Check sheet for the modelled part. Datum: model origin and axes. Units: mm. Face numbers are marked on the shaded views. A direction names the side the tool comes from. Coordinates: 2 decimals unless noted, no trailing zeros. Order: outer loops, then holes, each group sorted by start corner. A loop starts at its lowest first (then second) coordinate and runs counter-clockwise, first axis right, second up.
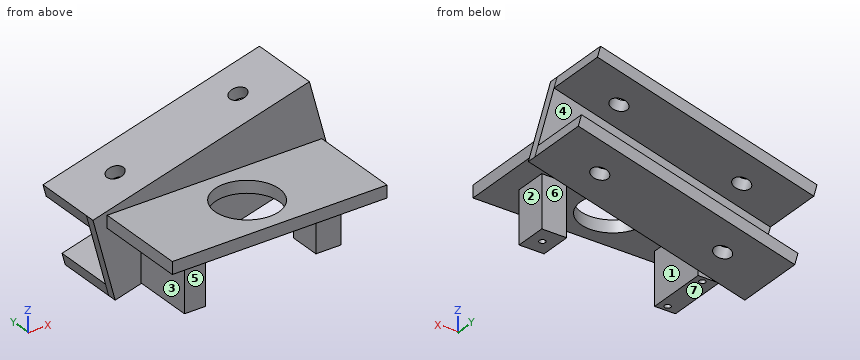
from build123d import *

# Parameters (mm, degrees)
SKETCH1_W           = 70
SKETCH1_H           = 30
SKETCH1_R           = 10.5
BOSS_EXTRUDE1_DEPTH = 4
SKETCH3_W           = 8.150987667
SKETCH3_H           = 10.43538234
SKETCH3_W_2         = 6.820916115
SKETCH3_H_2         = 20
BOSS_EXTRUDE2_DEPTH = 17
SKETCH4_R           = 1
CUT_EXTRUDE1_DEPTH  = 17
BOSS_EXTRUDE4_DEPTH = 3
BOSS_EXTRUDE5_DEPTH = 20
SKETCH10_R          = 2.75
CUT_EXTRUDE2_DEPTH  = 47.267747797


with BuildPart() as part:
    # Sketch1 → Boss-Extrude1 (new body)
    with BuildSketch(Plane.XY):
        with Locations((35, -15)):
            Rectangle(SKETCH1_W, SKETCH1_H)
        with Locations((35, -15)):
            Circle(SKETCH1_R, mode=Mode.SUBTRACT)
    extrude(amount=BOSS_EXTRUDE1_DEPTH)

    # Sketch3 → Boss-Extrude2 (add)
    with BuildSketch(Plane(origin=(0, 0, 0), x_dir=(-1, 0, 0), z_dir=(0, 0, -1))):
        with Locations((-58.424506167, -14.156074174)):
            Rectangle(SKETCH3_W, SKETCH3_H)
        with Locations((-10.910458058, -15)):
            Rectangle(SKETCH3_W_2, SKETCH3_H_2)
    extrude(amount=BOSS_EXTRUDE2_DEPTH)

    # Sketch4 → Cut-Extrude1 (cut)
    with BuildSketch(Plane(origin=(0, 0, -17), x_dir=(-1, 0, 0), z_dir=(0, 0, -1))):
        with Locations((-58.5, -14.289099526)):
            Circle(SKETCH4_R)
        with Locations((-11.5, -7)):
            Circle(SKETCH4_R)
        with Locations((-11.5, -23)):
            Circle(SKETCH4_R)
    extrude(amount=-CUT_EXTRUDE1_DEPTH, mode=Mode.SUBTRACT)

    # Sketch7 → Boss-Extrude4 (add)
    with BuildSketch(Plane(origin=(0, 0, 0), x_dir=(1, 0, 0), z_dir=(0, 1, 0))):
        Polygon((-4.630368757, -4), (65.950788783, -22.912164164), (73.197722046, 4.133758972), (2.616564506, 23.045923136), align=None)
    extrude(amount=BOSS_EXTRUDE4_DEPTH)

    # Sketch9 → Boss-Extrude5 (add)
    with BuildSketch(Plane(origin=(0, 3, 0), x_dir=(1, 0, 0), z_dir=(0, 1, 0))):
        Polygon((-4.630368757, -4), (65.950788783, -22.912164164), (66.943950204, -19.205635281), (-3.595092577, -0.136296695), align=None)
        Polygon((2.616564506, 23.045923136), (1.581288325, 19.182219831), (72.162445865, 0.270055667), (73.197722046, 4.133758972), align=None)
    extrude(amount=BOSS_EXTRUDE5_DEPTH)

    # Sketch10 → Cut-Extrude2 (cut, through all)
    with BuildSketch(Plane(origin=(5.936757371, 0, -22.156280139), x_dir=(-0.965925826, 0, -0.258819045), z_dir=(0.258819045, 0, -0.965925826))):
        with Locations((-53.953749554, 11.5)):
            Circle(SKETCH10_R)
        with Locations((-12.488324975, 11.5)):
            Circle(SKETCH10_R)
    extrude(amount=-CUT_EXTRUDE2_DEPTH, mode=Mode.SUBTRACT)


solid = part.part
(1) Go/stop test with flat-tipped pins: P1, Ø10, axis at x = 39.5, y = -3, coming from the -Z side; P2, Ø13.5, axis at y = -19, z = -12, coming from the -X side; P3, Ø1.6, axis at x = 11.5, y = -7, coming from the +Z side; P4, Ø1.5, axis at x = 23, z = -18, coming from the +Y side. Record where each tip stops, or that it passes through.
Filled in:
P1: stops at z = -14.23
P2: stops at x = 7.5
P3: stops at z = 4
P4: stops at y = 23
(2) Cross-section at B-B (z = -11.5). Enter the section's corners in (x, y), and give its area (3 significant figures).
Filled in:
outline: (-0.48, 0) - (45.71, 0) - (45.71, 23) - (30.25, 23) - (30.25, 3) - (-0.48, 3) - close; (7.5, -25) - (14.32, -25) - (14.32, -5) - (7.5, -5) - close; (54.35, -19.37) - (62.5, -19.37) - (62.5, -8.94) - (54.35, -8.94) - close; hole circle Ø2 at (11.5, -23); hole circle Ø2 at (11.5, -7); hole circle Ø2 at (58.5, -14.29)
area: 660 mm2
(3) Cross-section at D-D (y = -23). Enter the section's corners in (x, z), and give its area (3 significant figures).
Filled in:
outline: (0, 0) - (7.5, 0) - (7.5, -17) - (10.5, -17) - (10.5, 0) - (12.5, 0) - (12.5, -17) - (14.32, -17) - (14.32, 0) - (28.2, 0) - (28.2, 4) - (0, 4) - close; (41.8, 0) - (70, 0) - (70, 4) - (41.8, 4) - close
area: 308 mm2
(4) Cross-section at C-C (x = 35). Enter the section's corners in (y, z), and give its area (3 significant figures).
Filled in:
outline: (-30, 0) - (-25.5, 0) - (-25.5, 4) - (-30, 4) - close; (-4.5, 0) - (0, 0) - (0, -14.37) - (23, -14.37) - (23, -10.23) - (3, -10.23) - (3, 10.57) - (23, 10.57) - (23, 14.62) - (0, 14.62) - (0, 4) - (-4.5, 4) - close
area: 287 mm2
(5) Thickness scan on probe 1 along Y at (x, z) = (11.5, -4); probe 2 along X at (y, z) = (-10.5, -3.5); probe 3 along Y at (x, z) = (58, -7). Record the ranges inside material, lowest first.
Filled in:
probe 1: y = -25 to -24, -22 to -8, -6 to -5, 0 to 3
probe 2: x = 7.5 to 14.32, 54.35 to 62.5
probe 3: y = -19.37 to -15.16, -13.42 to -8.94, 0 to 8.76, 14.24 to 23
(6) Release check for a two-part mould opening along Y. For the marked faces 4, 5, 6 and 7 record: +Y half, -Y half, draft (parallel to the pull), parting line (faces both ways), or undercut.
Filled in:
face 4: +Y half
face 5: -Y half
face 6: undercut
face 7: draft
(7) Tool access check on the marked faces 1, 2 and 3. Record the directions out of +Z, -Z, +X, -X, +Y, -Y that give a thin tool (end or side, any length) a straight path to the whole face; none if there is none.
Filled in:
face 1: -Z, -Y
face 2: -Z, +X, -Y
face 3: -Z, -X, -Y
(8) Cross-section at A-A (y = 7.5). Enter the section's corners in (x, z), and give its area (3 significant figures).
Filled in:
outline: (-4.63, 4) - (-3.6, 0.14) - (66.94, 19.21) - (65.95, 22.91) - close; (1.58, -19.18) - (2.62, -23.05) - (73.2, -4.13) - (72.16, -0.27) - close
area: 579 mm2
